For this review, take the finished solid that the model builds, in its own axes (mm). A direction names the side the tool comes from. Give positions to 0.01 mm unless a question says otherwise; leave off trailing zeros. Loops run counter-clockwise (first coordinate to the right, second up) from the corner with the lowest first, then second, coordinate; pieces in that order, holes last.
```python
from build123d import *

# Parameters (mm, degrees)
SKETCH1_W           = 82
SKETCH1_H           = 56
BOSS_EXTRUDE1_DEPTH = 15
SKETCH3_W           = 80
SKETCH3_H           = 54
CUT_EXTRUDE1_DEPTH  = 3
CUT_EXTRUDE2_DEPTH  = 10
SKETCH5_W           = 60
SKETCH5_H           = 2
CUT_EXTRUDE3_DEPTH  = 11


with BuildPart() as part:
    # Sketch1 → Boss-Extrude1 (new body)
    with BuildSketch(Plane(origin=(0, 0, 0), x_dir=(1, 0, 0), z_dir=(0, 1, 0))):
        with Locations((41, 28)):
            Rectangle(SKETCH1_W, SKETCH1_H)
    extrude(amount=BOSS_EXTRUDE1_DEPTH)

    # Sketch3 → Cut-Extrude1 (cut)
    with BuildSketch(Plane(origin=(0, 15, 0), x_dir=(1, 0, 0), z_dir=(0, 1, 0))):
        with Locations((41, 28)):
            Rectangle(SKETCH3_W, SKETCH3_H)
    extrude(amount=-CUT_EXTRUDE1_DEPTH, mode=Mode.SUBTRACT)

    # 3DSketch1 → Cut-Extrude2 (cut)
    with BuildSketch(Plane(origin=(80, 12, -2), x_dir=(-0.8320502943378438, 0, -0.554700196225229), z_dir=(0, 1, 0))):
        Polygon((0, 0), (28.844410204, -43.266615306), (93.744333162, 0), (64.899922958, 43.266615306), align=None)
    extrude(amount=-CUT_EXTRUDE2_DEPTH, mode=Mode.SUBTRACT)

    # Sketch5 → Cut-Extrude3 (cut)
    with BuildSketch(Plane.XZ):
        with Locations((41, -5)):
            Rectangle(SKETCH5_W, SKETCH5_H)
        with Locations((41, -51)):
            Rectangle(SKETCH5_W, SKETCH5_H)
        with BuildLine():
            Line((70.653805937, -23), (70.653805937, -25.5))
            ThreePointArc((70.653805937, -25.5), (73.153805937, -28), (70.653805937, -30.5))
            Line((70.653805937, -30.5), (70.653805937, -33))
            ThreePointArc((70.653805937, -33), (68.153805937, -35.5), (65.653805937, -33))
            Line((65.653805937, -33), (65.653805937, -23))
            ThreePointArc((65.653805937, -23), (68.153805937, -20.5), (70.653805937, -23))
        make_face()
    extrude(amount=-CUT_EXTRUDE3_DEPTH, mode=Mode.SUBTRACT)


solid = part.part
```
Item 1: For L1, parallel to Z at x = 23, y = 0.75; L2, parallel to Z at x = 37, y = 4.25; L3, parallel to X at y = 8, z = -25, list the stretches that pass through material, from the lowest coordinate up.
Answer:
L1: z = -56 to -52, -50 to -6, -4 to 0
L2: z = -56 to -54, -2 to 0
L3: x = 0 to 2, 80 to 82
Item 2: Clearance check with a flat-ended pin moving along its axis: pin 1 Ø10 at (x, z) = (15, -10) entering from +Y. State where the tip first meets the part, or that it passes through.
Answer:
pin 1: stops at y = 2
Item 3: Take a section at A-A on z = -28. Give the boundary of the cut face in (x, y).
Answer:
outline: (0, 0) - (65.65, 0) - (65.65, 2) - (2, 2) - (2, 12) - (1, 12) - (1, 15) - (0, 15) - close; (73.15, 0) - (82, 0) - (82, 15) - (81, 15) - (81, 12) - (80, 12) - (80, 2) - (73.15, 2) - close
Item 4: Take a section at C-C on x = 56.5. Give the boundary of the cut face in (y, z), and give its area (3 significant figures).
Answer:
outline: (0, -56) - (15, -56) - (15, -55) - (12, -55) - (12, -54) - (2, -54) - (2, -52) - (0, -52) - close; (0, -50) - (2, -50) - (2, -6) - (0, -6) - close; (0, -4) - (2, -4) - (2, -2) - (12, -2) - (12, -1) - (15, -1) - (15, 0) - (0, 0) - close
area: 150 mm2
Item 5: Take a section at D-D on y = 14. Give the boundary of the cut face in (x, z).
Answer:
outline: (0, -56) - (82, -56) - (82, 0) - (0, 0) - close; hole (1, -55) - (81, -55) - (81, -1) - (1, -1) - close
Item 6: Take a section at B-B on y = 8.75. Give the boundary of the cut face in (x, z), and give its area (3 significant figures).
Answer:
outline: (0, -56) - (82, -56) - (82, 0) - (0, 0) - close; hole (2, -54) - (80, -54) - (80, -2) - (2, -2) - close
area: 536 mm2
Item 7: Tool access review of faces 1 (the cylindrical face through (68.2, 1, -35.5)), 2 (the flat face through (40, 0, -28)), 3 (the flat face through (80, 7, -28)): name each direction out of +Z, -Z, +X, -X, +Y, -Y from which nothing blocks a thin tool from reaching the whole face with its end or side.
Answer:
face 1: +Y, -Y
face 2: +Z, -Z, +X, -X, -Y
face 3: +Y
Item 8: The part is to be moulded in two halves that separate along Z. For faces 4 (the flat face through (0, 7, -28)), 5 (the cylindrical face through (73.153, 0.986, -27.945)), 6 (the flat face through (41, 1, -52)), 7 (the flat face through (40, 7, -56)), say which applies: released by +Z, released by -Z, zero draft, split by the parting line, or undercut.
Answer:
face 4: zero draft
face 5: undercut
face 6: undercut
face 7: released by -Z
